from build123d import *

# Parameters (mm, degrees)
SKETCH_1_R          = 7.5
EXTRUDE_1_DEPTH     = 50
EXTRUDE_START       = -10
EXTRUDE_2_DEPTH     = 10
SKETCH_3_R          = 5
SKETCH_3_R_2        = 1.75
CUT_EXTRUDE_1_DEPTH = 10
SKETCH_4_W          = 44
SKETCH_4_H          = 22
CUT_EXTRUDE_2_DEPTH = 50
SKETCH_5_W          = 48
SKETCH_5_H          = 58
EXTRUDE_3_DEPTH     = 20
SKETCH_6_R          = 4
CUT_EXTRUDE_3_DEPTH = 50
SKETCH_7_W          = 10
SKETCH_7_H          = 32
CUT_EXTRUDE_4_DEPTH = 50
SKETCH_8_R          = 1.5
CUT_EXTRUDE_5_DEPTH = 20


with BuildPart() as part:
    # 草图1 → 凸台-拉伸1 (new body)
    with BuildSketch(Plane(origin=(0, 0, 0), x_dir=(1, 0, 0), z_dir=(0, 1, 0))):
        with BuildLine():
            Line((-11, 0), (-11, -11))
            Line((-11, -11), (11, -11))
            Line((11, -11), (11, 0))
            ThreePointArc((11, 0), (0, 11), (-11, 0))
        make_face()
        with Locations(Location((0, 0, 0), (0, 0, 270))):
            Circle(SKETCH_1_R, mode=Mode.SUBTRACT)
    extrude(amount=EXTRUDE_1_DEPTH)

    # 草图2 → 凸台-拉伸2 (add)
    with BuildSketch(Plane(origin=(0, 50, 0), x_dir=(1, 0, 0), z_dir=(0, 1, 0)).offset(EXTRUDE_START)):
        with BuildLine():
            Line((-11, 11), (0, 11))
            ThreePointArc((0, 11), (-7.778174593, 7.778174593), (-11, 0))
            Line((-11, 0), (-11, -11))
            Line((-11, -11), (-33, -11))
            Line((-33, -11), (-33, 6))
            ThreePointArc((-33, 6), (-31.535533906, 9.535533906), (-28, 11))
            Line((-28, 11), (-11, 11))
        make_face()
    extrude(amount=EXTRUDE_2_DEPTH)

    # 草图3 → 切除-拉伸1 (cut)
    with BuildSketch(Plane(origin=(0, 50, 0), x_dir=(1, 0, 0), z_dir=(0, 1, 0))):
        with Locations(Location((-22, 0, 0), (0, 0, 270))):
            Circle(SKETCH_3_R)
        with Locations(Location((-27.656854249, 5.656854249, 0), (0, 0, 270))):
            Circle(SKETCH_3_R_2)
        with Locations(Location((-16.343145751, 5.656854249, 0), (0, 0, 270))):
            Circle(SKETCH_3_R_2)
        with Locations(Location((-16.343145751, -5.656854249, 0), (0, 0, 270))):
            Circle(SKETCH_3_R_2)
        with Locations(Location((-27.656854249, -5.656854249, 0), (0, 0, 270))):
            Circle(SKETCH_3_R_2)
    extrude(amount=-CUT_EXTRUDE_1_DEPTH, mode=Mode.SUBTRACT)

    # 镜向1: part across plane


with BuildPart() as part_1:
    add(part.part)
    add(part.part.mirror(Plane(origin=(11, 50, 11), x_dir=(0, 0, 1), z_dir=(-1, 0, 0))))

    # 草图4 → 切除-拉伸2 (cut)
    with BuildSketch(Plane.XZ):
        with Locations((-11, 0)):
            Rectangle(SKETCH_4_W, SKETCH_4_H)
    extrude(amount=-CUT_EXTRUDE_2_DEPTH, mode=Mode.SUBTRACT)

    # 草图5 → 凸台-拉伸3 (add)
    with BuildSketch(Plane.XY.offset(11)):
        with Locations((35, 21)):
            Rectangle(SKETCH_5_W, SKETCH_5_H)
    extrude(amount=EXTRUDE_3_DEPTH)

    # 草图6 → 切除-拉伸3 (cut)
    with BuildSketch(Plane(origin=(59, 0, 0), x_dir=(0, 0, -1), z_dir=(1, 0, 0))):
        with Locations(Location((-21, 43.5, 0), (0, 0, 90))):
            Circle(SKETCH_6_R)
        with Locations(Location((-21, -1.5, 0), (0, 0, 90))):
            Circle(SKETCH_6_R)
    extrude(amount=-CUT_EXTRUDE_3_DEPTH, mode=Mode.SUBTRACT)

    # 草图7 → 切除-拉伸4 (cut)
    with BuildSketch(Plane(origin=(59, 0, 0), x_dir=(0, 0, -1), z_dir=(1, 0, 0))):
        with Locations((-21, 21)):
            Rectangle(SKETCH_7_W, SKETCH_7_H)
    extrude(amount=-CUT_EXTRUDE_4_DEPTH, mode=Mode.SUBTRACT)

    # 草图8 → 切除-拉伸5 (cut)
    with BuildSketch(Plane(origin=(0, 0, 11), x_dir=(-1, 0, 0), z_dir=(0, 0, -1))):
        with Locations((-50, 21.08)):
            Circle(SKETCH_8_R)
    extrude(amount=-CUT_EXTRUDE_5_DEPTH, mode=Mode.SUBTRACT)


solid = part_1.part
Work out the finished part from the listing and answer in its coordinate system (mm). A direction names the side the tool comes from. Round coordinates to 2 decimals unless told otherwise and drop trailing zeros. Write each loop counter-clockwise with the first axis right and the second up, starting at its lowest first coordinate (ties: lowest second). Pieces come first, ordered by that corner, then holes. Notation, with made-up numbers: (53, -8) - (95, -8) arc R18 cw to (95, 26) - close; hole circle Ø11 at (-23.75, 71). An arc over 180 degrees is marked (long way). Answer in a Markdown table with one row per item. Add a question column.
1. A cutting plane is placed at D-D, the plane z = 21. Determine the outline of the cut face in (x, y), and give its area (3 significant figures).
2. A cutting plane is placed at A-A, the plane y = 7. Determine the outline of the cut face in (x, z), and give its area (3 significant figures).
3. The mould has two halves that part along Z. Classify faces 1 (the flat face through (35, 50, 14)), 2 (the cylindrical face through (22, 25, -11)), 3 (the flat face through (35, 37, 21)): +Z half, -Z half, draft (parallel to the pull), parting line (faces both ways), or undercut.
4. Given pin 1 (6 mm diameter, centred on x = 44, z = 0, fed in from +Y); pin 2 (24 mm diameter, centred on x = 37, z = -4.5, fed in from -Y); pin 3 (5.5 mm diameter, centred on y = 13, z = 5, fed in from +X); pin 4 (1.5 mm diameter, centred on x = 35, y = 4, fed in from -Z), each flat-ended and moving along its own axis, determine where each tip first touches the part or whether it passes through.
5. Find the intervals of material crossed by line 1 along X through (y, z) = (42, 0); line 2 along Y through (x, z) = (50, 29); line 3 along X through (y, z) = (21, 27), in increasing order. Write a range as from..to.
6. For faces 4 (the flat face through (24.6, 0, 7.2)), 5 (the flat face through (11, 21, 12)), 6 (the flat face through (33, 20, 5)), 7 (the flat face through (35, 5, 21)), determine the directions among +Z, -Z, +X, -X, +Y, -Y from which every point of the face is accessible in a straight line to the end or side of a thin tool.
7. A cutting plane is placed at B-B, the plane y = 21.08. Determine the outline of the cut face in (x, z).
8. A cutting plane is placed at C-C, the plane x = 17. Determine the outline of the cut face in (y, z), and give its area (3 significant figures).
Worked out:
| question | item | result |
|---|---|---|
| 1 | outline | (11, -8) - (59, -8) - (59, -5.5) - (11, -5.5) - close; (11, 2.5) - (59, 2.5) - (59, 5) - (11, 5) - close; (11, 37) - (59, 37) - (59, 39.5) - (11, 39.5) - close; (11, 47.5) - (59, 47.5) - (59, 50) - (11, 50) - close |
| 1 | area | 480 mm^2 |
| 2 | outline | (11, 0) arc R11 ccw to (33, 0) - (33, 11) - (59, 11) - (59, 16) - (11, 16) - close; (11, 26) - (59, 26) - (59, 31) - (11, 31) - close; hole circle Ø15 at (22, 0) |
| 2 | area | 735 mm^2 |
| 3 | face 1 | draft |
| 3 | face 2 | -Z half |
| 3 | face 3 | undercut |
| 4 | pin 1 | through |
| 4 | pin 2 | y = 0 |
| 4 | pin 3 | x = 33 |
| 4 | pin 4 | z = 11 |
| 5 | line 1 | 11..14.5, 29.5..39, 49..55 |
| 5 | line 2 | -8..19.58, 22.58..50 |
| 5 | line 3 | 11..48.5, 51.5..59 |
| 6 | face 4 | -Z, +X, -X, -Y |
| 6 | face 5 | +Z, -Z, -X, +Y, -Y |
| 6 | face 6 | -Z, +X, -Y |
| 6 | face 7 | +X, -X |
| 7 | outline | (11, 0) arc R11 ccw to (33, 0) - (33, 11) - (48.5, 11) - (48.5, 16) - (11, 16) - close; (11, 26) - (48.5, 26) - (48.5, 31) - (11, 31) - close; (51.5, 11) - (59, 11) - (59, 16) - (51.5, 16) - close; (51.5, 26) - (59, 26) - (59, 31) - (51.5, 31) - close; hole circle Ø15 at (22, 0) |
| 8 | outline | (-8, 11) - (0, 11) - (0, 5.59) - (50, 5.59) - (50, 31) - (-8, 31) - close; (0, -9.8) - (50, -9.8) - (50, -5.59) - (0, -5.59) - close; hole circle Ø8 at (-1.5, 21); hole (5, 16) - (37, 16) - (37, 26) - (5, 26) - close; hole circle Ø8 at (43.5, 21) |
| 8 | area | 1,220 mm^2 |
